Print and shaded views of the part. All mm, measured from the part's lowest x, y and z. Coordinates: 2 decimals unless noted, no trailing zeros. Loops run counter-clockwise (first coordinate to the right, second up) from the corner with the lowest first, then second, coordinate; pieces in that order, holes last.
1) Saw through at D-D, the plane z = 206. Write the cut outline in (x, y) (1 decimal).
2) Saw through at A-A, the plane z = 162.5. Write the cut outline in (x, y) (1 decimal).
3) Pin check, flat tips, straight feed: pin 1 Ø1.6 at (x, y) = (165.5, 1.5) entering from -Z; pin 2 Ø1 at (x, y) = (174, 2) entering from +Z. Stop position of each tip, or through.
4) Wall check: line 1 along Z through (x, y) = (169, 2.4); line 2 along Z through (x, y) = (17.5, 1.9); line 3 along X through (y, z) = (0.1, 195). Give the ranges that are in metal, low to high.
5) Saw through at B-B, the plane x = 37. Give the number of separate pieces and of enclosed holes in the cut face, and give its area (3 significant figures).
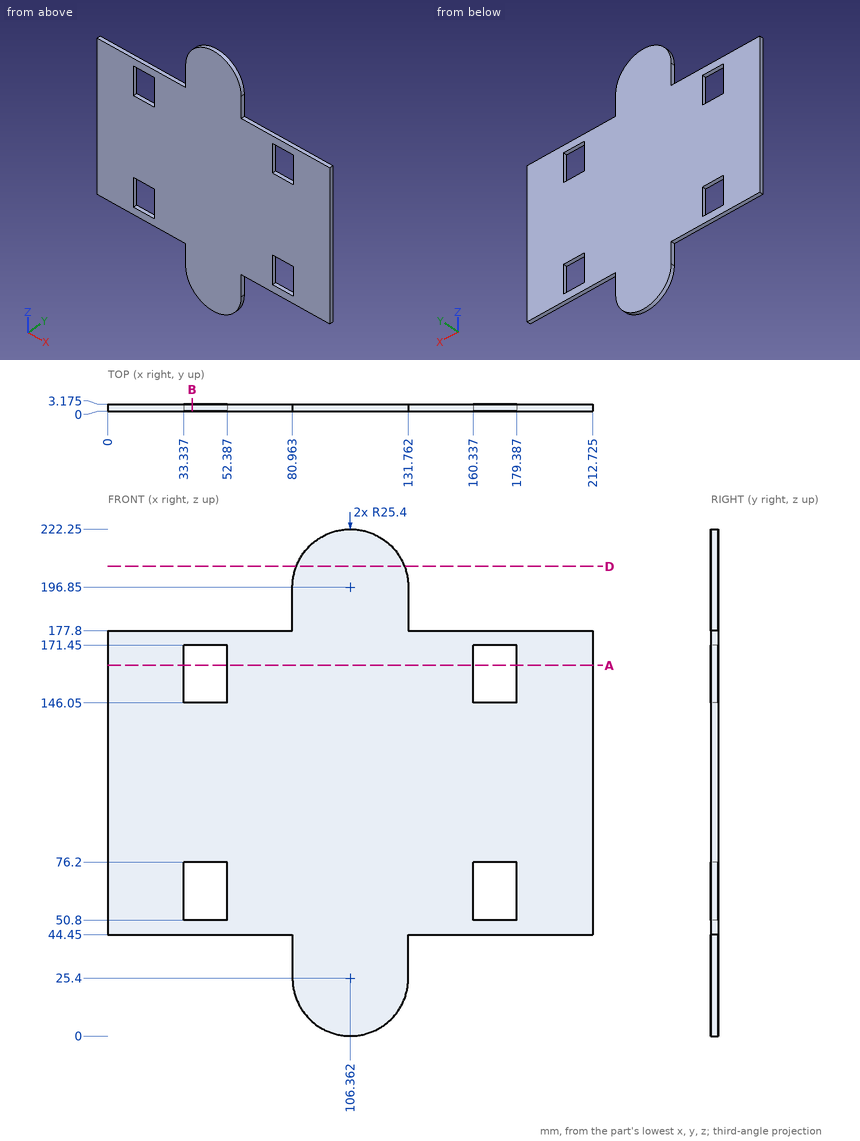
Data:
1. outline: (82.7, 0) - (130.1, 0) - (130.1, 3.2) - (82.7, 3.2) - close
2. outline: (0, 0) - (33.3, 0) - (33.3, 3.2) - (0, 3.2) - close; (52.4, 0) - (160.3, 0) - (160.3, 3.2) - (52.4, 3.2) - close; (179.4, 0) - (212.7, 0) - (212.7, 3.2) - (179.4, 3.2) - close
3. pin 1: stops at z = 44.45
3. pin 2: stops at z = 177.8
4. line 1: z = 44.45 to 50.8, 76.2 to 146.05, 171.45 to 177.8
4. line 2: z = 44.45 to 177.8
4. line 3: x = 80.96 to 131.76
5. separate pieces: 3
5. enclosed holes: 0
5. area: 262 mm2
